Source: CAD feature listing. Evaluate the final solid. Frame: model axes, mm. A direction names the side the tool comes from. Coordinates: 2 decimals unless noted, no trailing zeros. Loops run counter-clockwise (first coordinate to the right, second up) from the corner with the lowest first, then second, coordinate; pieces in that order, holes last.
Item 1: Pull-direction query (X, two-part tool) for faces 6 (the flat face through (-14.75, 18, 0)), 7 (the flat face through (17.75, 17, 0)), 8 (the flat face through (0, 1, -5)); classes: +X half, -X half, draft (parallel to the pull), parting line (faces both ways), or undercut.
Item 2: Reachability of faces 1 (the cylindrical face through (16.27, 33.47, 0.46)), 2 (the cylindrical face through (-16.27, 28.47, -0.46)), 3 (the flat face through (14.75, 19, 0)), 4 (the flat face through (-17.75, 18, 0)), 5 (the flat face through (0, 0, 0)) from +Z, -Z, +X, -X, +Y, -Y: full face, straight path, thin tool, end or side. Return the list, or none.
Item 3: Section query C-C, the plane y = 7.5. Return the cut outline in (x, z), then the cut area to 3 significant figures.
Item 4: Line query: probe 1 along X at (y, z) = (13, -1); probe 2 along Y at (x, z) = (16.1, 0); probe 3 along Y at (x, z) = (-12.5, -2.5). Output: solid intervals per line, ascending.
Item 5: Section query A-A, the plane y = 25. Return the cut outline in (x, z), then the cut area to 3 significant figures.
Item 6: Pin query (flat end, axial travel): pin 1 Ø5 at (x, z) = (-4.5, 0.5) entering from +Y; pin 2 Ø4 at (x, y) = (14, 21.5) entering from -Z. Return the tip coordinate at first contact, or that it passes through.
Item 7: Section query B-B, the plane z = 0. Return the cut outline in (x, y).
Item 8: Section query D-D, the plane z = -2.25. Return the cut outline in (x, y), then the cut area to 3 significant figures.
```python
from build123d import *

# Parameters (mm, degrees)
BOSS_EXTRUDE1_DEPTH = 5
SKETCH2_R           = 3.5
CUT_EXTRUDE1_DEPTH  = 5
CUT_EXTRUDE2_REACH  = 52.102
SKETCH3_R           = 3.5


with BuildPart() as part:
    # Sketch1 → Boss-Extrude1 (new, symmetric)
    with BuildSketch(Plane.XY):
        Polygon((14.75, 2), (-14.75, 2), (-14.75, 35), (-17.75, 35), (-17.75, 0), (17.75, 0), (17.75, 35), (14.75, 35), align=None)
    extrude(amount=BOSS_EXTRUDE1_DEPTH, both=True)

    # Sketch2 → Cut-Extrude1 (cut, symmetric)
    with BuildSketch(Plane(origin=(17.75, 0, 0), x_dir=(0, 0, -1), z_dir=(1, 0, 0))):
        with Locations((0, 30)):
            Circle(SKETCH2_R)
    extrude(amount=CUT_EXTRUDE1_DEPTH, both=True, mode=Mode.SUBTRACT)

    # Sketch3 → Cut-Extrude2 (cut, up to next)
    with BuildSketch(Plane.ZY.offset(17.75), mode=Mode.PRIVATE) as cut_extrude2_sk1:
        with Locations((0, 25)):
            Circle(SKETCH3_R)
    cut_extrude2_tool1 = extrude(cut_extrude2_sk1.sketch, amount=-CUT_EXTRUDE2_REACH, mode=Mode.PRIVATE) & part.part
    add(cut_extrude2_tool1.solids().sort_by_distance((-17.75, 25, 0))[0], mode=Mode.SUBTRACT)


solid = part.part
```
Verdict:
1. face 6: undercut
1. face 7: +X half
1. face 8: draft
2. face 1: +X
2. face 2: -X
2. face 3: +Z, -Z, +Y
2. face 4: +Z, -Z, -X, +Y, -Y
2. face 5: +Z, -Z, +X, -X, -Y
3. outline: (-17.75, -5) - (-14.75, -5) - (-14.75, 5) - (-17.75, 5) - close; (14.75, -5) - (17.75, -5) - (17.75, 5) - (14.75, 5) - close
3. area: 60.0 mm2
4. probe 1: x = -17.75 to -14.75, 14.75 to 17.75
4. probe 2: y = 0 to 26.5, 33.5 to 35
4. probe 3: y = 0 to 2
5. outline: (-17.75, -5) - (-14.75, -5) - (-14.75, -3.5) - (-17.75, -3.5) - close; (-17.75, 3.5) - (-14.75, 3.5) - (-14.75, 5) - (-17.75, 5) - close; (14.75, -5) - (17.75, -5) - (17.75, 5) - (14.75, 5) - close
5. area: 39.0 mm2
6. pin 1: stops at y = 2
6. pin 2: stops at z = -5
7. outline: (-17.75, 0) - (17.75, 0) - (17.75, 26.5) - (14.75, 26.5) - (14.75, 2) - (-14.75, 2) - (-14.75, 21.5) - (-17.75, 21.5) - close; (-17.75, 28.5) - (-14.75, 28.5) - (-14.75, 35) - (-17.75, 35) - close; (14.75, 33.5) - (17.75, 33.5) - (17.75, 35) - (14.75, 35) - close
8. outline: (-17.75, 0) - (17.75, 0) - (17.75, 27.32) - (14.75, 27.32) - (14.75, 2) - (-14.75, 2) - (-14.75, 22.32) - (-17.75, 22.32) - close; (-17.75, 27.68) - (-14.75, 27.68) - (-14.75, 35) - (-17.75, 35) - close; (14.75, 32.68) - (17.75, 32.68) - (17.75, 35) - (14.75, 35) - close
8. area: 237 mm2
